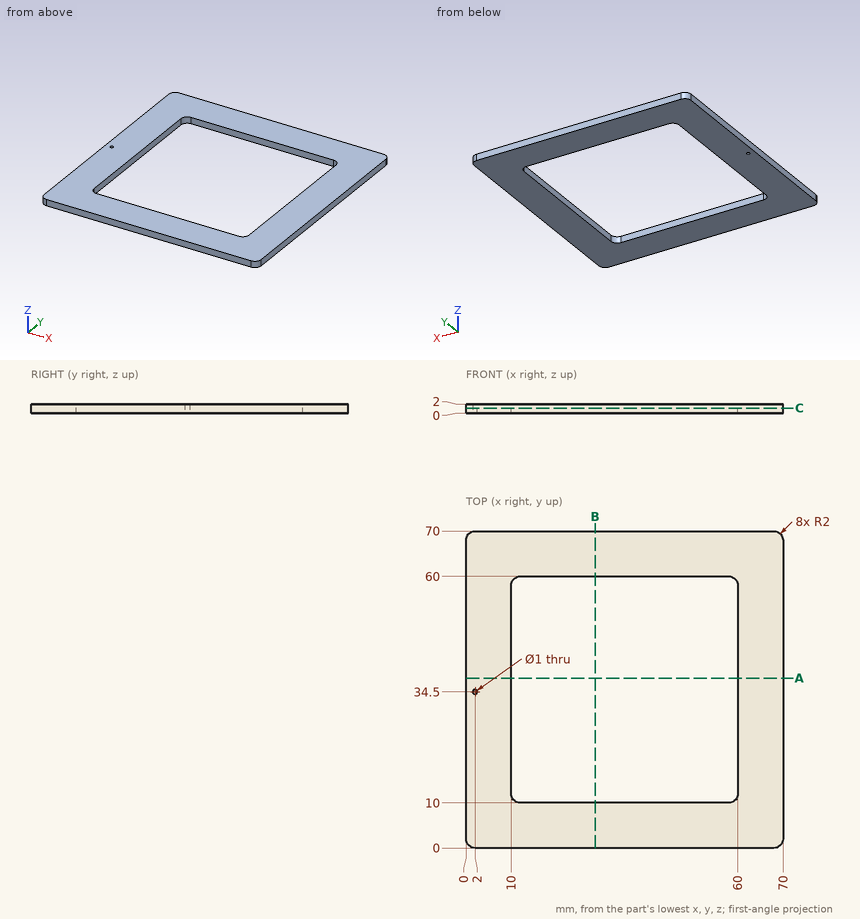
Print and shaded views of the part. All mm, measured from the part's lowest x, y and z. Give positions to 0.01 mm unless a question says otherwise; leave off trailing zeros. Write each loop counter-clockwise with the first axis right and the second up, starting at its lowest first coordinate (ties: lowest second). Pieces come first, ordered by that corner, then holes. Notation, with made-up numbers: (-39, 83) -> (-11, 83) arc R8 cw to (-11, 98) -> close; hole circle Ø9 at (-12.5, 22.25). An arc over 180 degrees is marked (long way). Use CSV: the item, a comma, the result in double quotes. Start each with the question number.
1) Drill centre lines: L1, parallel to X at y = 27, z = 1.4; L2, parallel to X at y = 34.5, z = 1.3. Where is each one in solid material? Low to high.
2) Cut at A-A on y = 37.5. List the corners of the cut face in (x, z), plus the area to 3 significant figures.
3) Cut at C-C on z = 1.1. List the corners of the cut face in (x, y).
Final values:
1,L1,"x = 0 to 10, 60 to 70"
1,L2,"x = 0 to 1.5, 2.5 to 10, 60 to 70"
2,outline,"(0, 0) -> (10, 0) -> (10, 2) -> (0, 2) -> close; (60, 0) -> (70, 0) -> (70, 2) -> (60, 2) -> close"
2,area,"40.0 mm2"
3,outline,"(0, 2) arc R2 ccw to (2, 0) -> (68, 0) arc R2 ccw to (70, 2) -> (70, 68) arc R2 ccw to (68, 70) -> (2, 70) arc R2 ccw to (0, 68) -> close; hole circle Ø1 at (2, 34.5); hole (10, 12) arc R2 ccw to (12, 10) -> (58, 10) arc R2 ccw to (60, 12) -> (60, 58) arc R2 ccw to (58, 60) -> (12, 60) arc R2 ccw to (10, 58) -> close"
